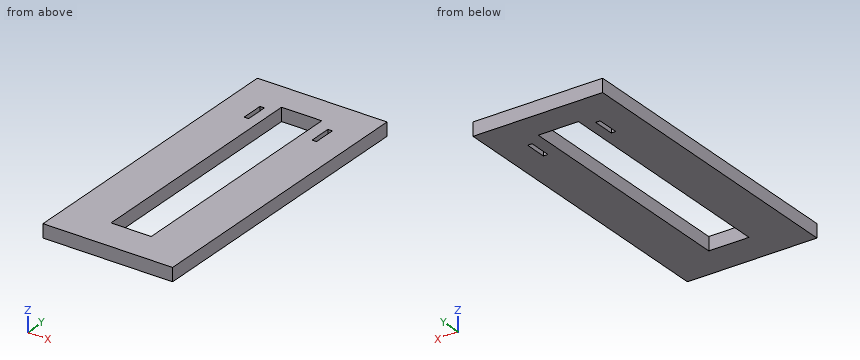
```python
from build123d import *

# Parameters (mm, degrees)
F0_W     = 127
F0_H     = 686.889625
F0_W_2   = 12.7
F0_H_2   = 63.5
F0_H_3   = 93.98
F0_W_3   = 114.3
F0_H_4   = 82.730375
F1_DEPTH = 38.1


with BuildPart() as f1:
    # F0 (on Top) → F1 (new body)
    with BuildSketch(Plane.XY):
        with Locations((-59.372775, 4.420739)):
            Rectangle(F0_W, F0_H)
        with Locations((-32.702775, 290.258352)):
            Rectangle(F0_W_2, F0_H_2, mode=Mode.SUBTRACT)
        with Locations((-59.372775, -386.014073)):
            Rectangle(F0_W, F0_H_3)
        with Locations((61.277225, -386.014073)):
            Rectangle(F0_W_3, F0_H_3)
        with Locations((181.927225, -386.014073)):
            Rectangle(F0_W, F0_H_3)
        with Locations((181.927225, 4.420739)):
            Rectangle(F0_W, F0_H)
        with Locations((160.337225, 290.258352)):
            Rectangle(F0_W_2, F0_H_2, mode=Mode.SUBTRACT)
        with Locations((181.927225, 389.230739)):
            Rectangle(F0_W, F0_H_4)
        with Locations((61.277225, 389.230739)):
            Rectangle(F0_W_3, F0_H_4)
        with Locations((-59.372775, 389.230739)):
            Rectangle(F0_W, F0_H_4)
    extrude(amount=F1_DEPTH)


solid = f1.part
```
Part model, mm, in its own coordinate system. Round coordinates to 2 decimals unless told otherwise and drop trailing zeros. Loops run counter-clockwise (first coordinate to the right, second up) from the corner with the lowest first, then second, coordinate; pieces in that order, holes last.
1. Slice it at B-B (y = 275.5). Give the cut face in (x, z), and give its area (3 significant figures).
Solutions:
outline: (-122.87, 0) - (-39.05, 0) - (-39.05, 38.1) - (-122.87, 38.1) - close; (-26.35, 0) - (4.13, 0) - (4.13, 38.1) - (-26.35, 38.1) - close; (118.43, 0) - (153.99, 0) - (153.99, 38.1) - (118.43, 38.1) - close; (166.69, 0) - (245.43, 0) - (245.43, 38.1) - (166.69, 38.1) - close
area: 8,710 mm2
2. Drill centre lines: line 1 along X through (y, z) = (292, 7.5); line 2 along Y through (x, z) = (155, 27); line 3 along X through (y, z) = (253, 13). Where is each one in solid material? Low to high.
Solutions:
line 1: x = -122.87 to -39.05, -26.35 to 4.13, 118.43 to 153.99, 166.69 to 245.43
line 2: y = -433 to 258.51, 322.01 to 430.6
line 3: x = -122.87 to 4.13, 118.43 to 245.43
3. Slice it at A-A (x = 67). Give the cut face in (y, z).
Solutions:
outline: (-433, 0) - (-339.02, 0) - (-339.02, 38.1) - (-433, 38.1) - close; (347.87, 0) - (430.6, 0) - (430.6, 38.1) - (347.87, 38.1) - close
4. Slice it at C-C (z = 11.5). Give the cut face in (x, y), and give its area (3 significant figures).
Solutions:
outline: (-122.87, -433) - (245.43, -433) - (245.43, 430.6) - (-122.87, 430.6) - close; hole (-39.05, 258.51) - (-26.35, 258.51) - (-26.35, 322.01) - (-39.05, 322.01) - close; hole (4.13, -339.02) - (118.43, -339.02) - (118.43, 347.87) - (4.13, 347.87) - close; hole (153.99, 258.51) - (166.69, 258.51) - (166.69, 322.01) - (153.99, 322.01) - close
area: 238,000 mm2
5. Slice it at D-D (y = -59). Give the cut face in (x, z).
Solutions:
outline: (-122.87, 0) - (4.13, 0) - (4.13, 38.1) - (-122.87, 38.1) - close; (118.43, 0) - (245.43, 0) - (245.43, 38.1) - (118.43, 38.1) - close
